Part print with two shaded views. Sizes in mm from the minimum x, y, z corner. A direction names the side the tool comes from. Round coordinates to 2 decimals unless told otherwise and drop trailing zeros. Loops run counter-clockwise (first coordinate to the right, second up) from the corner with the lowest first, then second, coordinate; pieces in that order, holes last. Notation, with made-up numbers: (26.5, -33) -> (49.5, -33) arc R31 cw to (49.5, 0) -> close; hole circle Ø8 at (22.25, -7). An arc over 180 degrees is marked (long way). Answer as a JSON object with one key per item and string values. Group by question number.
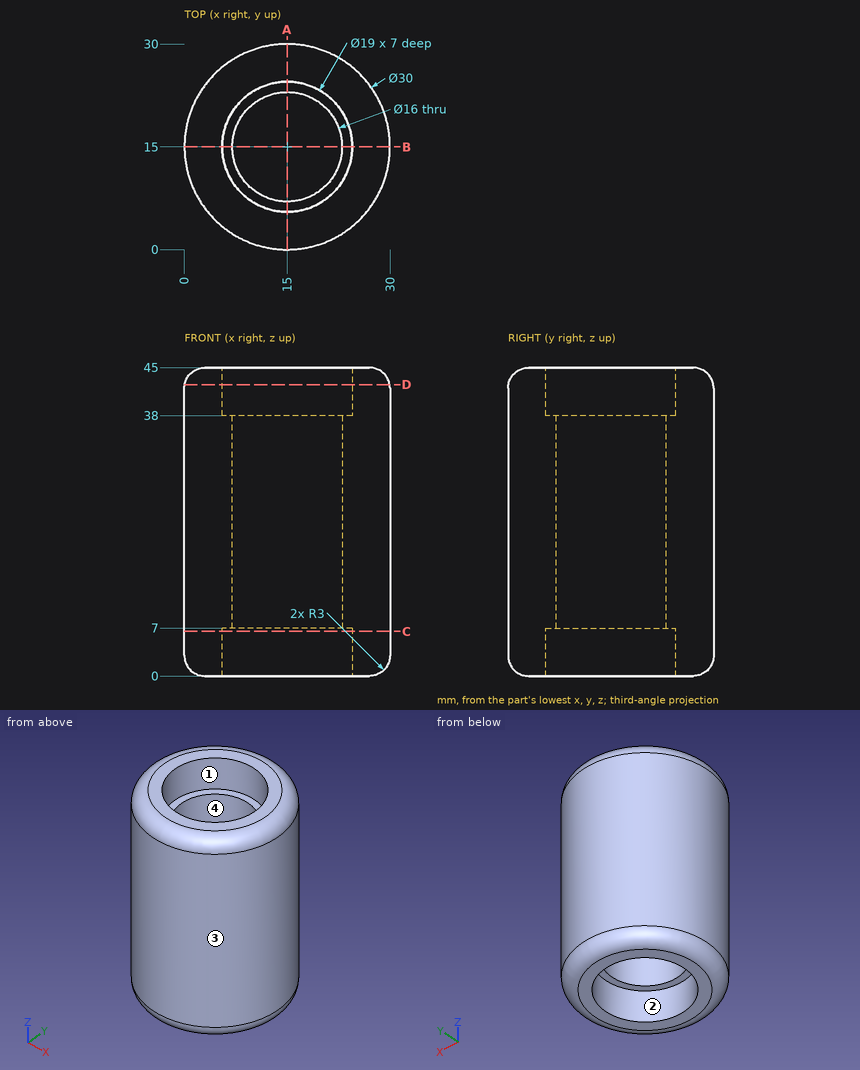
Item 1: Band-saw the part on C-C, the plane z = 6.5. List the corners of the cut face in (x, y), plus the area to 3 significant figures.
Item 2: Drill centre lines: line 1 (Y direction, x = 15, z = 4.75); line 2 (Y direction, x = 15, z = 29.5); line 3 (Z direction, x = 19.5, y = 6.75). Where is each one in solid material? Low to high.
Item 3: Band-saw the part on A-A, the plane x = 15. List the corners of the cut face in (y, z).
Item 4: Drop flat-ended pins along their axis: pin 1 Ø6 at (x, z) = (4, 15.5) entering from -Y; pin 2 Ø10 at (y, z) = (23, 21) entering from -X; pin 3 Ø13 at (x, y) = (15, 15) entering from +Z; pin 4 Ø3 at (x, y) = (24.5, 26.5) entering from +Z. Give the stop position or say it passes through.
Item 5: Which spindle directions (+Z, -Z, +X, -X, +Y, -Y) get a long thin tool onto all of the face, cutting with end or side? Do the marked faces 1 and 2. Say none if no direction does.
Item 6: Band-saw the part on D-D, the plane z = 42.5. List the corners of the cut face in (x, y).
Item 7: Two-plate mould, pull along X, no slides. Class the marked faces 3 and 4: pulls with the +X half, pulls with the -X half, needs draft (parallel to the pull), parting line crosses it, or undercut.
Entries:
{
 "1": {"outline": "circle Ø30 at (15, 15); hole circle Ø19 at (15, 15)", "area": "423 mm²"},
 "2": {"line 1": "0 to 5.5, 24.5 to 30", "line 2": "0 to 7, 23 to 30", "line 3": "7 to 38"},
 "3": {"outline": "(0, 3) arc R3 ccw to (3, 0) -> (5.5, 0) -> (5.5, 7) -> (7, 7) -> (7, 38) -> (5.5, 38) -> (5.5, 45) -> (3, 45) arc R3 ccw to (0, 42) -> close; (23, 7) -> (24.5, 7) -> (24.5, 0) -> (27, 0) arc R3 ccw to (30, 3) -> (30, 42) arc R3 ccw to (27, 45) -> (24.5, 45) -> (24.5, 38) -> (23, 38) -> close"},
 "4": {"pin 1": "y = 2.31", "pin 2": "x = 0.3", "pin 3": "through", "pin 4": "z = 44.64"},
 "5": {"face 1": "+Z", "face 2": "-Z"},
 "6": {"outline": "circle Ø29.92 at (15, 15); hole circle Ø19 at (15, 15)"},
 "7": {"face 3": "parting line crosses it", "face 4": "undercut"}
}
